```python
from build123d import *

# Parameters (mm, degrees)
SKETCH1_R           = 1
BOSS_EXTRUDE1_DEPTH = 1.5


with BuildPart() as part:
    # Sketch1 → Boss-Extrude1 (new body)
    with BuildSketch(Plane(origin=(0, 0, 0), x_dir=(1, 0, 0), z_dir=(0, 1, 0))):
        with BuildLine():
            Line((-0.4136064, 2.465548569), (-0.143377771, 3.149767964))
            Line((-0.143377771, 3.149767964), (0.143377771, 3.149767964))
            Line((0.143377771, 3.149767964), (0.4136064, 2.465548569))
            ThreePointArc((0.4136064, 2.465548569), (0.519779227, 2.445369002), (0.6249807, 2.420619575))
            Line((0.6249807, 2.420619575), (1.150143936, 2.935773209))
            Line((1.150143936, 2.935773209), (1.41210816, 2.819139222))
            Line((1.41210816, 2.819139222), (1.380677197, 2.084161817))
            ThreePointArc((1.380677197, 2.084161817), (1.469463131, 2.022542486), (1.55550296, 1.957143465))
            Line((1.55550296, 1.957143465), (2.244795308, 2.214156596))
            Line((2.244795308, 2.214156596), (2.436672219, 2.001055698))
            Line((2.436672219, 2.001055698), (2.109016362, 1.342404553))
            ThreePointArc((2.109016362, 1.342404553), (2.165063509, 1.25), (2.217064626, 1.15525947))
            Line((2.217064626, 1.15525947), (2.951301179, 1.109692193))
            Line((2.951301179, 1.109692193), (3.039913515, 0.836971465))
            Line((3.039913515, 0.836971465), (2.472687439, 0.368533346))
            ThreePointArc((2.472687439, 0.368533346), (2.486304738, 0.261321158), (2.495275677, 0.153620618))
            Line((2.495275677, 0.153620618), (3.147500263, -0.186648072))
            Line((3.147500263, -0.186648072), (3.117526147, -0.471832738))
            Line((3.117526147, -0.471832738), (2.408808394, -0.669060624))
            ThreePointArc((2.408808394, -0.669060624), (2.377641291, -0.772542486), (2.342030895, -0.874580635))
            Line((2.342030895, -0.874580635), (2.799467958, -1.450715189))
            Line((2.799467958, -1.450715189), (2.656090187, -1.699052774))
            Line((2.656090187, -1.699052774), (1.928424495, -1.590967934))
            ThreePointArc((1.928424495, -1.590967934), (1.857862064, -1.672826516), (1.783827694, -1.75155895))
            Line((1.783827694, -1.75155895), (1.967382211, -2.463940471))
            Line((1.967382211, -2.463940471), (1.735392103, -2.63249115))
            Line((1.735392103, -2.63249115), (1.114598481, -2.237782435))
            ThreePointArc((1.114598481, -2.237782435), (1.016841608, -2.283863644), (0.91718448, -2.325676811))
            Line((0.91718448, -2.325676811), (0.795118206, -3.051128062))
            Line((0.795118206, -3.051128062), (0.51462896, -3.110747891))
            Line((0.51462896, -3.110747891), (0.108048264, -2.497664023))
            ThreePointArc((0.108048264, -2.497664023), (0, -2.5), (-0.108048264, -2.497664023))
            Line((-0.108048264, -2.497664023), (-0.51462896, -3.110747891))
            Line((-0.51462896, -3.110747891), (-0.795118206, -3.051128062))
            Line((-0.795118206, -3.051128062), (-0.91718448, -2.325676811))
            ThreePointArc((-0.91718448, -2.325676811), (-1.016841608, -2.283863644), (-1.114598481, -2.237782435))
            Line((-1.114598481, -2.237782435), (-1.735392103, -2.63249115))
            Line((-1.735392103, -2.63249115), (-1.967382211, -2.463940471))
            Line((-1.967382211, -2.463940471), (-1.783827694, -1.75155895))
            ThreePointArc((-1.783827694, -1.75155895), (-1.857862064, -1.672826516), (-1.928424495, -1.590967934))
            Line((-1.928424495, -1.590967934), (-2.656090187, -1.699052774))
            Line((-2.656090187, -1.699052774), (-2.799467958, -1.450715189))
            Line((-2.799467958, -1.450715189), (-2.342030895, -0.874580635))
            ThreePointArc((-2.342030895, -0.874580635), (-2.377641291, -0.772542486), (-2.408808394, -0.669060624))
            Line((-2.408808394, -0.669060624), (-3.117526147, -0.471832738))
            Line((-3.117526147, -0.471832738), (-3.147500263, -0.186648072))
            Line((-3.147500263, -0.186648072), (-2.495275677, 0.153620618))
            ThreePointArc((-2.495275677, 0.153620618), (-2.486304738, 0.261321158), (-2.472687439, 0.368533346))
            Line((-2.472687439, 0.368533346), (-3.039913515, 0.836971465))
            Line((-3.039913515, 0.836971465), (-2.951301179, 1.109692193))
            Line((-2.951301179, 1.109692193), (-2.217064626, 1.15525947))
            ThreePointArc((-2.217064626, 1.15525947), (-2.165063509, 1.25), (-2.109016362, 1.342404553))
            Line((-2.109016362, 1.342404553), (-2.436672219, 2.001055698))
            Line((-2.436672219, 2.001055698), (-2.244795308, 2.214156596))
            Line((-2.244795308, 2.214156596), (-1.55550296, 1.957143465))
            ThreePointArc((-1.55550296, 1.957143465), (-1.469463131, 2.022542486), (-1.380677197, 2.084161817))
            Line((-1.380677197, 2.084161817), (-1.41210816, 2.819139222))
            Line((-1.41210816, 2.819139222), (-1.150143936, 2.935773209))
            Line((-1.150143936, 2.935773209), (-0.6249807, 2.420619575))
            ThreePointArc((-0.6249807, 2.420619575), (-0.519779227, 2.445369002), (-0.4136064, 2.465548569))
        make_face()
        with Locations(Location((0, 0, 0), (0, 0, 270))):
            Circle(SKETCH1_R, mode=Mode.SUBTRACT)
    extrude(amount=BOSS_EXTRUDE1_DEPTH)


solid = part.part
```
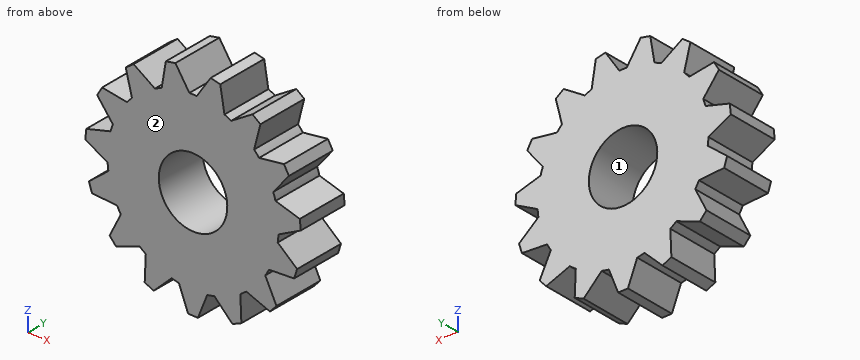
Model file for the job. Use its own axes, mm. Face numbers are marked on the shaded views. Round coordinates to 2 decimals unless told otherwise and drop trailing zeros. Order: outer loops, then holes, each group sorted by start corner. A loop starts at its lowest first (then second) coordinate and runs counter-clockwise, first axis right, second up. Notation, with made-up numbers: (-18, 11.25) -> (3, 11.25) arc R26 cw to (3, 29.25) -> close; hole circle Ø11 at (-23, 86). An arc over 180 degrees is marked (long way). Use one line per item in the form item = value.
Item 1: Drill centre lines: line 1 (X direction, y = 0.8, z = 0); line 2 (Z direction, x = 2, y = 0.9); line 3 (X direction, y = 1.4, z = 1.25). Where is each one in solid material? Low to high.
Returned:
line_1 = -2.79 to -1, 1 to 2.79
line_2 = -2.12 to 1.6
line_3 = -2.64 to 2.64
Item 2: Cut at A-A, the plane x = 0. Write the cut outline in (y, z), and give its area (3 significant figures).
Returned:
outline = (0, -3.15) -> (1.5, -3.15) -> (1.5, -1) -> (0, -1) -> close; (0, 1) -> (1.5, 1) -> (1.5, 2.5) -> (0, 2.5) -> close
area = 5.47 mm^2
Item 3: Cut at B-B, the plane z = -0.25. Write the cut outline in (x, y).
Returned:
outline = (-2.49, 0) -> (-0.97, 0) -> (-0.97, 1.5) -> (-2.49, 1.5) -> close; (0.97, 0) -> (2.49, 0) -> (2.49, 1.5) -> (0.97, 1.5) -> close
Item 4: Pull direction X, two halves, no side cores. Call the marked faces 1 and 2: released by +X, released by -X, zero draft, split by the parting line, or undercut.
Returned:
face_1 = undercut
face_2 = zero draft
